from build123d import *

# Parameters (mm, degrees)
F1_DEPTH = 28.4
F3_DEPTH = 71.3
F4_W     = 6.577678
F4_H     = 17.057187
F5_DEPTH = 70.5


with BuildPart() as f1:
    # F0 (on Front) → F1 (new body, symmetric)
    with BuildSketch(Plane.XZ):
        Polygon((19.129556, 18.970141), (-42.722672, 18.970141), (-42.722672, -30.288463), (-22.955466, -30.288463), (-22.955466, -21.042513), (25.824901, -21.042513), (25.824901, -30.288463), (54.519232, -30.288463), (95.488362, -30.288463), (95.488362, 35.549089), (62.292963, 35.549089), (44.954456, 8.130061), (44.954456, 4.941802), (29.172573, 4.941802), (29.172573, 8.130061), align=None)
    extrude(amount=F1_DEPTH, both=True)

    # F2 (on face) → F3 (cut)
    with BuildSketch(Plane(origin=(-42.722672, 0, 0), x_dir=(0, -1, 0), z_dir=(-1, 0, 0))):
        Polygon((14.665993, 18.970141), (-12.753037, 18.970141), (-18.013665, 11.637147), (19.926621, 11.637147), align=None)
    extrude(amount=-F3_DEPTH, mode=Mode.SUBTRACT)

    # F4 (on face) → F5 (cut)
    with BuildSketch(Plane.XY.offset(11.637147)):
        with Locations((-39.433833, -1.036185)):
            Rectangle(F4_W, F4_H)
    extrude(amount=-F5_DEPTH, mode=Mode.SUBTRACT)


solid = f1.part
The model under review builds one solid part; all positions refer to its coordinate system, in mm. A direction names the side the tool comes from. Give positions to 0.01 mm unless a question says otherwise; leave off trailing zeros. Loops run counter-clockwise (first coordinate to the right, second up) from the corner with the lowest first, then second, coordinate; pieces in that order, holes last. Notation, with made-up numbers: (52, -39) -> (92, -39) arc R32 cw to (92, -9) -> close; hole circle Ø2 at (-25, 24). An arc over 180 degrees is marked (long way). Answer as a JSON object with one key per item and string values. Group by question number.
Q1. Insertion check: pin 1 (1.5 mm diameter, centred on x = -2.5, y = 2, fed in from -Z); pin 2 (12.5 mm diameter, centred on x = -3, y = 24.5, fed in from +Z); pin 3 (4.5 mm diameter, centred on x = 38, y = 11.5, fed in from +Z). Each pin has a flat end and moves straight along its axis. Give the tip position at first contact, or say it passes through.
Q2. Take a section at D-D (x = 12). Write out the cut boundary in (y, z).
Q3. Draft analysis for pull direction Z (two halves, no side actions). For faces 5 (the flat face through (79, 0, 35.549)), 6 (the flat face through (25.825, 0, -26)), 7 (the flat face through (-8.88, 15.35, 15.35)), state which applies: pulls with the +Z half, pulls with the -Z half, needs draft (parallel to the pull), parting line crosses it, or undercut.
Q4. Take a section at B-B (y = 9). Write out the cut boundary in (x, z).
Q5. Tool access review of faces 1 (the flat face through (29.173, 0, 7)), 2 (the flat face through (-8.9, -17.3, 15.3)), 3 (the flat face through (-39, -9.565, -9)), 4 (the flat face through (-11, -22, 18.97)): name each direction out of +Z, -Z, +X, -X, +Y, -Y from which nothing blocks a thin tool from reaching the whole face with its end or side.
Q6. Take a section at C-C (y = -18). Write out the cut boundary in (x, z), plus the area to 3 significant figures.
Q7. Take a section at A-A (x = -26.5). Write out the cut boundary in (y, z).
Q8. Wall thickness on line 1 along X through (y, z) = (6.5, 7.5) (3 decimals); line 2 along X through (y, z) = (-19, -26.5); line 3 along Z through (x, y) = (10, -12): over which ranges is each line inside the solid? List them lowest first.
Answer below:
{
 "1": {"pin 1": "stops at z = -21.04", "pin 2": "stops at z = 18.97", "pin 3": "stops at z = 4.94"},
 "2": {"outline": "(-28.4, -21.04) -> (28.4, -21.04) -> (28.4, 18.97) -> (12.75, 18.97) -> (18.01, 11.64) -> (-19.93, 11.64) -> (-14.67, 18.97) -> (-28.4, 18.97) -> close"},
 "3": {"face 5": "pulls with the +Z half", "face 6": "needs draft", "face 7": "undercut"},
 "4": {"outline": "(-42.72, -30.29) -> (-22.96, -30.29) -> (-22.96, -21.04) -> (25.82, -21.04) -> (25.82, -30.29) -> (95.49, -30.29) -> (95.49, 35.55) -> (62.29, 35.55) -> (44.95, 8.13) -> (44.95, 4.94) -> (29.17, 4.94) -> (29.17, 8.13) -> (25.92, 11.64) -> (-42.72, 11.64) -> close"},
 "5": {"face 1": "+Z, +Y, -Y", "face 2": "-X", "face 3": "+Z, -Z, -X", "face 4": "+Z, -X, +Y, -Y"},
 "6": {"outline": "(-42.72, -30.29) -> (-22.96, -30.29) -> (-22.96, -21.04) -> (25.82, -21.04) -> (25.82, -30.29) -> (95.49, -30.29) -> (95.49, 35.55) -> (62.29, 35.55) -> (44.95, 8.13) -> (44.95, 4.94) -> (29.17, 4.94) -> (29.17, 8.13) -> (25.92, 11.64) -> (-42.72, 11.64) -> close; (-42.72, 14.32) -> (23.44, 14.32) -> (19.13, 18.97) -> (-42.72, 18.97) -> close", "area": "6,500 mm2"},
 "7": {"outline": "(-28.4, -30.29) -> (28.4, -30.29) -> (28.4, 18.97) -> (12.75, 18.97) -> (18.01, 11.64) -> (-19.93, 11.64) -> (-14.67, 18.97) -> (-28.4, 18.97) -> close"},
 "8": {"line 1": "x = -36.145 to 29.173, 44.954 to 95.488", "line 2": "x = -42.72 to -22.96, 25.82 to 95.49", "line 3": "z = -21.04 to 11.64"}
}
